Verification items for the finished model (mm, model axes). A direction names the side the tool comes from. Coordinates: 2 decimals unless noted, no trailing zeros. Order: outer loops, then holes, each group sorted by start corner. A loop starts at its lowest first (then second) coordinate and runs counter-clockwise, first axis right, second up.
Q1. Depth check by flat-ended pin: P1, Ø16.5, axis at y = 5.5, z = 22, coming from the -X side; P2, Ø6.5, axis at x = 84.5, y = 4.5, coming from the +Z side; P3, Ø12.5, axis at x = -90, z = 17.5, coming from the +Y side; P4, Ø4, axis at y = 0, z = 19.68, coming from the -X side. Enter the tip coordinate at first touch or a pass-through.
Q2. Set-up check for faces 4 (the flat face through (12.7, 0, 16)), 5 (the cylindrical face through (-78.8, -0.41, 22.83)), 6 (the flat face through (87, 12.7, 7)): record each of +Z, -Z, +X, -X, +Y, -Y from which the full face is reachable in a straight line by a thin tool's end or side.
Q3. Draft check along X on faces 1 (the flat face through (-101.07, 0, 16)), 2 (the flat face through (-6.35, 0, 16)), 3 (the flat face through (-79, 0, 28.575)). Enter one of: pulls with the +X half, pulls with the -X half, needs draft (parallel to the pull), parting line crosses it, or undercut.
Q4. Thickness scan on line 1 (X direction, y = -5, z = 7.25); line 2 (X direction, y = 9, z = 11.5). Record the ranges inside material, lowest first.
Q5. Cross-section at A-A, the plane x = -89. Record the boundary of the cut face in (y, z) (3 decimals).
Q6. Cross-section at C-C, the plane x = -37. Record the boundary of the cut face in (y, z) (3 decimals), and give its area (3 significant figures).
Q7. Cross-section at B-B, the plane y = -7. Record the boundary of the cut face in (x, z) (3 decimals).
from build123d import *

# Parameters (mm, degrees)
F0_W     = 254
F0_H     = 50.8
F1_DEPTH = 3.175
F2_W     = 25.4
F2_H     = 25.4
F3_DEPTH = 25.4
F4_W     = 12.7
F4_H     = 20.3732
F4_H_2   = 40.7416
F5_W     = 12.7
F5_H     = 20.3708
F6_DEPTH = 38.1
F7_R     = 3.175
F8_DEPTH = 227.187036


with BuildPart() as f1:
    # F0 (on Top) → F1 (new body)
    with BuildSketch(Plane.XY):
        Rectangle(F0_W, F0_H)
    extrude(amount=F1_DEPTH)

    # F2 (on face) → F3 (join)
    with BuildSketch(Plane.XY.offset(3.175)):
        with Locations((-88.369727, 0)):
            Rectangle(F2_W, F2_H)
        Rectangle(F2_W, F2_H)
        with Locations((87.486036, 0)):
            Rectangle(F2_W, F2_H)
    extrude(amount=F3_DEPTH)

    # F4 (on face) + F5 (on face) → F6 (cut)
    with BuildSketch(Plane.XZ.offset(12.7)):
        with Locations((-88.369727, 38.7616)):
            Rectangle(F4_W, F4_H)
        with Locations((-88.369727, 18.3884)):
            Rectangle(F4_W, F4_H)
        with Locations((0, 28.575)):
            Rectangle(F4_W, F4_H_2)
    with BuildSketch(Plane.XZ.offset(12.7)):
        with Locations((87.486036, 38.7604)):
            Rectangle(F5_W, F5_H)
        with Locations((87.486036, 18.3896)):
            Rectangle(F5_W, F5_H)
    extrude(amount=-F6_DEPTH, mode=Mode.SUBTRACT)

    # F7 (on face) → F8 (cut, through all)
    with BuildSketch(Plane.YZ.offset(100.186036)):
        with Locations((0, 19.681644)):
            Circle(F7_R)
    extrude(amount=-F8_DEPTH, mode=Mode.SUBTRACT)


solid = f1.part
Check values:
1. P1: stops at x = -101.07
1. P2: stops at z = 8.2
1. P3: stops at y = 12.7
1. P4: passes through
2. face 4: +Z, +Y, -Y
2. face 5: +X, -X
2. face 6: +Z, +X, -X, +Y
3. face 1: pulls with the -X half
3. face 2: undercut
3. face 3: needs draft
4. line 1: x = -101.07 to -75.67, -12.7 to 12.7, 74.79 to 100.19
4. line 2: x = -101.07 to -94.72, -82.02 to -75.67, -12.7 to -6.35, 6.35 to 12.7, 74.79 to 81.14, 93.84 to 100.19
5. outline: (-25.4, 0) - (25.4, 0) - (25.4, 3.175) - (12.7, 3.175) - (12.7, 8.202) - (-12.7, 8.202) - (-12.7, 3.175) - (-25.4, 3.175) - close
6. outline: (-25.4, 0) - (25.4, 0) - (25.4, 3.175) - (-25.4, 3.175) - close
6. area: 161 mm2
7. outline: (-127, 0) - (127, 0) - (127, 3.175) - (100.186, 3.175) - (100.186, 28.575) - (93.836, 28.575) - (93.836, 8.204) - (81.136, 8.204) - (81.136, 28.575) - (74.786, 28.575) - (74.786, 3.175) - (12.7, 3.175) - (12.7, 28.575) - (6.35, 28.575) - (6.35, 8.204) - (-6.35, 8.204) - (-6.35, 28.575) - (-12.7, 28.575) - (-12.7, 3.175) - (-75.67, 3.175) - (-75.67, 28.575) - (-82.02, 28.575) - (-82.02, 8.202) - (-94.72, 8.202) - (-94.72, 28.575) - (-101.07, 28.575) - (-101.07, 3.175) - (-127, 3.175) - close
